Work out the finished part from the listing and answer in its coordinate system (mm). A direction names the side the tool comes from. Round coordinates to 2 decimals unless told otherwise and drop trailing zeros. Loops run counter-clockwise (first coordinate to the right, second up) from the corner with the lowest first, then second, coordinate; pieces in that order, holes last. Notation, with made-up numbers: M -29,-12 L 18,-12 A4 cw 18,-6 Z; hole C -8,4.25 d4. An arc over 180 degrees is marked long. One line per item, written item: value.
```python
from build123d import *

# Parameters (mm, degrees)
CROQUIS1_R              = 35
SALIENTE_EXTRUIR1_DEPTH = 145
CROQUIS2_R              = 27.5
CROQUIS3_R              = 27.5
SALIENTE_EXTRUIR2_DEPTH = 120
CROQUIS5_R              = 36.5
SALIENTE_EXTRUIR3_DEPTH = 7
CROQUIS4_R              = 23
CORTAR_EXTRUIR1_DEPTH   = 525
REDONDEO1_R             = 10
SALIENTE_EXTRUIR4_START = -7
CROQUIS6_R              = 29
CROQUIS6_R_2            = 23
SALIENTE_EXTRUIR4_DEPTH = 7
REDONDEO2_R             = 2
CROQUIS7_W              = 119.738645001
CROQUIS7_H              = 395.389304841
CORTAR_EXTRUIR2_DEPTH   = 93


with BuildPart() as part:
    # Croquis1 → Saliente-Extruir1 (new body)
    with BuildSketch(Plane(origin=(0, 0, 0), x_dir=(1, 0, 0), z_dir=(0, 1, 0))):
        with Locations(Location((0, 0, 0), (0, 0, 270))):
            Circle(CROQUIS1_R)
    extrude(amount=SALIENTE_EXTRUIR1_DEPTH)

    # Croquis2 → section 1 of recubrir1
    with BuildSketch(Plane(origin=(0, 220, 0), x_dir=(1, 0, 0), z_dir=(0, 1, 0)), mode=Mode.PRIVATE) as recubrir1_s1:
        Circle(CROQUIS2_R)
    # loft up to a face of the part (recubrir1)
    loft([Face(Wire([part.edges().sort_by_distance((25.51390196, 145, -23.959148708))[0]])), recubrir1_s1.sketch])

    # Croquis3 → Saliente-Extruir2 (add)
    with BuildSketch(Plane(origin=(0, 220, 0), x_dir=(1, 0, 0), z_dir=(0, 1, 0))):
        with Locations(Location((0, 0, 0), (0, 0, 270))):
            Circle(CROQUIS3_R)
    extrude(amount=SALIENTE_EXTRUIR2_DEPTH)

    # Croquis5 → Saliente-Extruir3 (add)
    with BuildSketch(Plane.XZ):
        with Locations(Location((0, 0, 0), (0, 0, 270))):
            Circle(CROQUIS5_R)
    extrude(amount=-SALIENTE_EXTRUIR3_DEPTH)

    # Croquis4 → Cortar-Extruir1 (cut)
    with BuildSketch(Plane.XZ):
        with Locations(Location((0, 0, 0), (0, 0, 270))):
            Circle(CROQUIS4_R)
    extrude(amount=-CORTAR_EXTRUIR1_DEPTH, mode=Mode.SUBTRACT)

    # Redondeo1
    # the kernel refuses this fillet: 10 mm, written as the material it adds along each edge
    with BuildSketch(Plane(origin=(0, 220, 0), x_dir=(0, 0, 1), z_dir=(1, 0, 0))) as redondeo1_piece_1:
        with BuildLine():
            CenterArc((27.5 + REDONDEO1_R, -REDONDEO1_R * 0.0498756211209), REDONDEO1_R, 174.289406863, 5.710593137)
            Line((27.5 + REDONDEO1_R * 0.00496280979001, REDONDEO1_R * 0.0496280979001), (27.5, 0))
            Line((27.5, 0), (27.5, -REDONDEO1_R * 0.0498756211209))
        make_face()
    revolve(axis=Axis((0, 220, 0), (0, -1, 0)))
    # the kernel refuses this fillet: 10 mm, written as the material it takes off along each edge
    with BuildSketch(Plane(origin=(0, 145, 0), x_dir=(0, 0, 1), z_dir=(-1, 0, 0))) as redondeo1_2_piece_1:
        with BuildLine():
            CenterArc((35 - REDONDEO1_R, -REDONDEO1_R * 0.0498756211209), REDONDEO1_R, 0, 5.710593137)
            Line((35 - REDONDEO1_R * 0.00496280979001, REDONDEO1_R * 0.0496280979001), (35, 0))
            Line((35, 0), (35, -REDONDEO1_R * 0.0498756211209))
        make_face()
    revolve(axis=Axis((0, 145, 0), (0, 1, 0)), mode=Mode.SUBTRACT)

    # Croquis6 → Saliente-Extruir4 (add)
    with BuildSketch(Plane(origin=(0, 340, 0), x_dir=(1, 0, 0), z_dir=(0, 1, 0)).offset(SALIENTE_EXTRUIR4_START)):
        with Locations(Location((0, 0, 0), (0, 0, 270))):
            Circle(CROQUIS6_R)
        with Locations(Location((0, 0, 0), (0, 0, 90))):
            Circle(CROQUIS6_R_2, mode=Mode.SUBTRACT)
    extrude(amount=SALIENTE_EXTRUIR4_DEPTH)

    # Redondeo2
    # the kernel refuses this fillet: 2 mm, written as the material it adds along each edge
    with BuildSketch(Plane(origin=(0, 7, 0), x_dir=(0, 0, 1), z_dir=(1, 0, 0))) as redondeo2_piece_1:
        with BuildLine():
            CenterArc((37, -1.936491673), REDONDEO2_R, 104.477512186, 75.522487814)
            Line((35, -1.936491673), (34.96, -1.936491673))
            Line((34.96, -1.936491673), (34.96, 0))
            Line((34.96, 0), (35, 0.04))
            ThreePointArc((35, 0.04), (35.75, 0.04), (36.49, 0.038729833))
            Line((36.49, 0.038729833), (36.5, 0))
        make_face()
    revolve(axis=Axis((0, 7, 0), (0, -1, 0)))
    # the kernel refuses this fillet: 2 mm, written as the material it takes off along each edge
    with BuildSketch(Plane(origin=(0, 333, 0), x_dir=(0, 0, 1), z_dir=(-1, 0, 0))) as redondeo2_2_piece_1:
        with BuildLine():
            CenterArc((27, 1.936491673), REDONDEO2_R, 284.477512186, 75.522487814)
            Line((29, 1.936491673), (29.04, 1.936491673))
            Line((29.04, 1.936491673), (29.04, 0))
            Line((29.04, 0), (29, -0.04))
            ThreePointArc((29, -0.04), (28.25, -0.04), (27.51, -0.038729833))
            Line((27.51, -0.038729833), (27.5, 0))
        make_face()
    revolve(axis=Axis((0, 333, 0), (0, 1, 0)), mode=Mode.SUBTRACT)

    # Croquis7 → Cortar-Extruir2 (cut)
    with BuildSketch(Plane(origin=(0, 0, 0), x_dir=(0, 0, -1), z_dir=(1, 0, 0))):
        with Locations((-9.607607261, 197.694652421)):
            Rectangle(CROQUIS7_W, CROQUIS7_H)
    extrude(amount=-CORTAR_EXTRUIR2_DEPTH, mode=Mode.SUBTRACT)


solid = part.part
```
1) For faces 1 (the face through (0, 135, 28)), 2 (the face through (27.493, 275.962, 0.605)), 3 (the face through (28.993, 337.433, 0.638)), determine the directions among +Z, -Z, +X, -X, +Y, -Y from which every point of the face is accessible in a straight line to the end or side of a thin tool.
Check values:
face 1: +Z, -Z, -X, +Y, -Y
face 2: +X
face 3: +X, +Y
2) Find section C-C (y = 66). Give the vertices of the cut face in (x, z).
Check values:
outline: M 0,-35 A35 ccw 0,35 L 0,23 A23 cw 0,-23 Z
3) The mould has two halves that part along Y. Classify faces 4 (the face through (23.2, 340, 2)), 5 (the face through (31.19, 183.02, 0.69)), 6 (the face through (27, 0, 1)), 7 (the face through (34.99, 75.77, 0.77)): +Y half, -Y half, draft (parallel to the pull), parting line (faces both ways), or undercut.
Check values:
face 4: +Y half
face 5: undercut
face 6: -Y half
face 7: draft
4) Each of these flat-tipped pins is pushed along its axis until it touches: pin 1 (4 mm diameter, centred on y = 232.5, z = 17.5, fed in from +X); pin 2 (2 mm diameter, centred on y = 53, z = -9.5, fed in from +X); pin 3 (2 mm diameter, centred on x = 13, y = 45.5, fed in from -Z); pin 4 (3 mm diameter, centred on x = 8.5, z = 19, fed in from -Y). Where does it stop, or does it pass through?
Check values:
pin 1: x = 22.72
pin 2: x = 33.95
pin 3: z = -32.88
pin 4: through
5) Find section B-B (y = 298). Give the vertices of the cut face in (x, z).
Check values:
outline: M 0,-27.5 A27.5 ccw 0,27.5 L 0,23 A23 cw 0,-23 Z
6) Find the intervals of material crossed by probe 1 along Z at (x, y) = (8, 289); probe 2 along Z at (x, y) = (17, 163); probe 3 along X at (y, z) = (18, 12.5), in increasing order. Write a range as from..to.
Check values:
probe 1: -26.31..-21.56, 21.56..26.31
probe 2: -28.52..-15.49, 15.49..28.52
probe 3: 19.31..32.69
7) Find section A-A (z = 0). Give the vertices of the cut face in (x, y), then the cut area to 3 significant figures.
Check values:
outline: M 23,0 L 36.5,0 L 36.5,7 A2 cw 35,8.94 L 35,144.5 A10 ccw 34.95,145.5 L 27.55,219.5 A10 cw 27.5,220.5 L 27.5,333 A2 ccw 29,334.94 L 29,340 L 23,340 Z
area: 2,920 mm2
